The listing builds one solid part. Answer for the finished solid, in the listing's coordinates (mm). A direction names the side the tool comes from. Give positions to 0.01 mm unless a question says otherwise; leave off trailing zeros. Loops run counter-clockwise (first coordinate to the right, second up) from the corner with the lowest first, then second, coordinate; pieces in that order, holes last. Notation, with made-up numbers: (38.5, 68.5) - (55.5, 68.5) arc R27 ccw to (55.5, 101.5) - close; hole circle Ø10 at (47, -33). An arc over 180 degrees is marked (long way). Answer in a Markdown table with one row per item. Add a question column.
```python
from build123d import *
from OCP.BRepFilletAPI import BRepFilletAPI_MakeChamfer

# Parameters (mm, degrees)
BOSS_EXTRUDE1_DEPTH   = 11.43
F_4_CLEARANCE_HOLE1_D = 3.2639
CUT_EXTRUDE1_DEPTH    = 29.112648399
CHAMFER1_SIZE         = 1.905
CHAMFER1_SIZE2        = 0.693363296


with BuildPart() as part:
    # Sketch1 → Boss-Extrude1 (new, symmetric)
    with BuildSketch(Plane.XY):
        Polygon((-19.05, 3.81), (-25.4, 3.81), (-25.4, -3.81), (25.4, -3.81), (25.4, 3.81), (19.05, 3.81), (19.05, 0), (-19.05, 0), align=None)
    extrude(amount=BOSS_EXTRUDE1_DEPTH, both=True)

    # #4 Clearance Hole1 (through all)
    with Locations(Plane(origin=(0, 3.81, 0), x_dir=(1, 0, 0), z_dir=(0, 1, 0))):
        with Locations((22.225, -6.35), (-22.225, 6.35), (-22.225, -6.35), (22.225, 6.35)):
            Hole(F_4_CLEARANCE_HOLE1_D / 2)

    # Sketch4 → Cut-Extrude1 (cut, through all)
    with BuildSketch(Plane(origin=(0, 0, 0), x_dir=(1, 0, 0), z_dir=(0, 1, 0))):
        with BuildLine():
            Line((17.78, -11.43), (17.78, 1.27))
            ThreePointArc((17.78, 1.27), (13.97, 5.08), (10.16, 1.27))
            Line((10.16, 1.27), (10.16, -11.43))
            Line((10.16, -11.43), (17.78, -11.43))
        make_face()
    extrude(amount=-CUT_EXTRUDE1_DEPTH, mode=Mode.SUBTRACT)

    # Chamfer1: one chamfer whose edges measure the first distance from different faces: ONE call of the kernel's chamfer builder (chamfer() names one face for all edges)
    chamfer1_edges_1 = [part.edges().sort_by_distance(p)[0] for p in [
        (19.05, 1.905, 11.43),
        (19.05, 1.905, -11.43),
    ]]
    chamfer1_side_1 = [part.faces().sort_by_distance(p)[0] for p in [
        (19.05, 1.905, 0),
    ]]
    chamfer1_edges_2 = [part.edges().sort_by_distance(p)[0] for p in [
        (-19.05, 1.905, -11.43),
        (-19.05, 1.905, 11.43),
    ]]
    chamfer1_side_2 = [part.faces().sort_by_distance(p)[0] for p in [
        (-19.05, 1.905, 0),
    ]]
    chamfer1_edges_3 = [part.edges().sort_by_distance(p)[0] for p in [
        (17.78, -1.905, 11.43),
    ]]
    chamfer1_side_3 = [part.faces().sort_by_distance(p)[0] for p in [
        (17.78, -1.905, 5.08),
    ]]
    chamfer1_edges_4 = [part.edges().sort_by_distance(p)[0] for p in [
        (10.16, -1.905, 11.43),
    ]]
    chamfer1_side_4 = [part.faces().sort_by_distance(p)[0] for p in [
        (10.16, -1.905, 5.08),
    ]]
    chamfer1 = BRepFilletAPI_MakeChamfer(part.part.solid().wrapped)
    for e in chamfer1_edges_1:
        chamfer1.Add(CHAMFER1_SIZE, CHAMFER1_SIZE2, e.wrapped, chamfer1_side_1[0].wrapped)  # the first distance lies on this face
    for e in chamfer1_edges_2:
        chamfer1.Add(CHAMFER1_SIZE, CHAMFER1_SIZE2, e.wrapped, chamfer1_side_2[0].wrapped)  # the first distance lies on this face
    for e in chamfer1_edges_3:
        chamfer1.Add(CHAMFER1_SIZE, CHAMFER1_SIZE2, e.wrapped, chamfer1_side_3[0].wrapped)  # the first distance lies on this face
    for e in chamfer1_edges_4:
        chamfer1.Add(CHAMFER1_SIZE, CHAMFER1_SIZE2, e.wrapped, chamfer1_side_4[0].wrapped)  # the first distance lies on this face
    add(Compound.cast(chamfer1.Shape()), mode=Mode.REPLACE)


solid = part.part
```
(1) Find the intervals of material crossed by line 1 along X through (y, z) = (0.75, 6.35); line 2 along X through (y, z) = (-1.5, 6.35); line 3 along X through (y, z) = (-0.5, -6.35), in increasing order. Write a range as [from, to].
(2) A cutting plane is placed at B-B on z = 6.35. Determine the outline of the cut face in (x, y), plus the area to 3 significant figures.
(3) A cutting plane is placed at A-A on y = 1.75. Determine the outline of the cut face in (x, z) (3 decimals), plus the area to 3 significant figures.
(4) Given pin 1 Ø3 at (x, z) = (-11.5, 3.5) entering from +Y; pin 2 Ø3 at (x, z) = (-22.225, -6.35) entering from -Y, each flat-ended and moving along its own axis, determine where each tip first touches the part or whether it passes through.
(5) A tool of negligible diameter and unlimited length cuts with its end or side. For faces 4 (the face through (0, -2, -11.43)), 5 (the face through (9.81, -1.88, 10.49)), 6 (the face through (19.05, 2, 0)), 7 (the face through (-19.4, 1.88, 10.49)), 8 (the face through (19.4, 1.93, -10.49)), from which of +Z, -Z, +X, -X, +Y, -Y can it reach the whole face along a straight path? Write none if from no direction.
(6) A cutting plane is placed at D-D on y = -3. Determine the outline of the cut face in (x, z) (3 decimals), plus the area to 3 significant figures.
(7) The mould has two halves that part along X. Classify faces 1 (the face through (20.67, -0.05, 5.86)), 2 (the face through (22, 3.81, 0)), 3 (the face through (-25.4, 0, 0)): pulls with the +X half, pulls with the -X half, needs draft (parallel to the pull), parting line crosses it, or undercut.
(8) A cutting plane is placed at C-C on z = -6.35. Determine the outline of the cut face in (x, y).
Evaluation:
| question | item | result |
|---|---|---|
| 1 | line 1 | x = [-25.4, -23.86], [-20.59, -19.05], [19.05, 20.59], [23.86, 25.4] |
| 1 | line 2 | x = [-25.4, -23.86], [-20.59, 10.16], [17.78, 20.59], [23.86, 25.4] |
| 1 | line 3 | x = [-25.4, -23.86], [-20.59, 20.59], [23.86, 25.4] |
| 2 | outline | (-25.4, -3.81) - (-23.86, -3.81) - (-23.86, 3.81) - (-25.4, 3.81) - close; (-20.59, -3.81) - (10.16, -3.81) - (10.16, 0) - (-19.05, 0) - (-19.05, 3.81) - (-20.59, 3.81) - close; (17.78, -3.81) - (20.59, -3.81) - (20.59, 3.81) - (19.05, 3.81) - (19.05, 0) - (17.78, 0) - close; (23.86, -3.81) - (25.4, -3.81) - (25.4, 3.81) - (23.86, 3.81) - close |
| 2 | area | 163 mm² |
| 3 | outline | (-25.4, -11.43) - (-19.743, -11.43) - (-19.05, -9.525) - (-19.05, 9.525) - (-19.743, 11.43) - (-25.4, 11.43) - close; (19.05, -9.525) - (19.743, -11.43) - (25.4, -11.43) - (25.4, 11.43) - (19.743, 11.43) - (19.05, 9.525) - close; hole circle Ø3.264 at (-22.225, -6.35); hole circle Ø3.264 at (-22.225, 6.35); hole circle Ø3.264 at (22.225, -6.35); hole circle Ø3.264 at (22.225, 6.35) |
| 3 | area | 254 mm² |
| 4 | pin 1 | stops at y = 0 |
| 4 | pin 2 | passes through |
| 5 | face 4 | -Z, +X, -X, +Y, -Y |
| 5 | face 5 | +Z, +Y, -Y |
| 5 | face 6 | +Z, -Z, +Y |
| 5 | face 7 | +Z, +Y |
| 5 | face 8 | -Z, +Y |
| 6 | outline | (-25.4, -11.43) - (25.4, -11.43) - (25.4, 11.43) - (18.473, 11.43) - (17.78, 9.525) - (17.78, -1.27) arc R3.81 cw to (10.16, -1.27) - (10.16, 9.525) - (9.467, 11.43) - (-25.4, 11.43) - close; hole circle Ø3.264 at (-22.225, -6.35); hole circle Ø3.264 at (-22.225, 6.35); hole circle Ø3.264 at (22.225, -6.35); hole circle Ø3.264 at (22.225, 6.35) |
| 6 | area | 1,010 mm² |
| 7 | face 1 | undercut |
| 7 | face 2 | needs draft |
| 7 | face 3 | pulls with the -X half |
| 8 | outline | (-25.4, -3.81) - (-23.86, -3.81) - (-23.86, 3.81) - (-25.4, 3.81) - close; (-20.59, -3.81) - (20.59, -3.81) - (20.59, 3.81) - (19.05, 3.81) - (19.05, 0) - (-19.05, 0) - (-19.05, 3.81) - (-20.59, 3.81) - close; (23.86, -3.81) - (25.4, -3.81) - (25.4, 3.81) - (23.86, 3.81) - close |
